from build123d import *

# Parameters (mm, degrees)
SKETCH_1_W          = 720
SKETCH_1_H          = 110
SKETCH_1_R          = 5
EXTRUDE_1_DEPTH     = 2
SKETCH_2_W          = 720
SKETCH_2_H          = 3
EXTRUDE_2_DEPTH     = 20
SKETCH_3_R          = 2.5
CUT_EXTRUDE_3_DEPTH = 114


with BuildPart() as part:
    # 草图1 → 凸台-拉伸1 (new body)
    with BuildSketch(Plane.XY):
        with Locations((266.780748393, 19.519407272)):
            Rectangle(SKETCH_1_W, SKETCH_1_H)
        with Locations((0, -5.480592728)):
            Circle(SKETCH_1_R, mode=Mode.SUBTRACT)
        with Locations((179.094970205, -5.480592728)):
            Circle(SKETCH_1_R, mode=Mode.SUBTRACT)
        with Locations((354.466526581, -5.480592728)):
            Circle(SKETCH_1_R, mode=Mode.SUBTRACT)
        with Locations((529.466526581, -5.480592728)):
            Circle(SKETCH_1_R, mode=Mode.SUBTRACT)
    extrude(amount=EXTRUDE_1_DEPTH)

    # 草图2 → 凸台-拉伸2 (add)
    with BuildSketch(Plane.XY.offset(2)):
        with Locations((266.780748393, 73.019407272)):
            Rectangle(SKETCH_2_W, SKETCH_2_H)
        with Locations((266.780748393, -33.980592728)):
            Rectangle(SKETCH_2_W, SKETCH_2_H)
    extrude(amount=EXTRUDE_2_DEPTH)

    # 草图3 → 切除-拉伸3 (cut)
    with BuildSketch(Plane(origin=(0, 74.519407272, 0), x_dir=(1, 0, 0), z_dir=(0, 1, 0))):
        with Locations(Location((456.780748393, -12, 0), (0, 0, 270))):
            Circle(SKETCH_3_R)
        with Locations(Location((616.780748393, -12, 0), (0, 0, 270))):
            Circle(SKETCH_3_R)
        with Locations(Location((436.780748393, -12, 0), (0, 0, 270))):
            Circle(SKETCH_3_R)
        with Locations(Location((276.780748393, -12, 0), (0, 0, 270))):
            Circle(SKETCH_3_R)
        with Locations(Location((256.780748393, -12, 0), (0, 0, 270))):
            Circle(SKETCH_3_R)
        with Locations(Location((96.780748393, -12, 0), (0, 0, 270))):
            Circle(SKETCH_3_R)
        with Locations(Location((76.780748393, -12, 0), (0, 0, 270))):
            Circle(SKETCH_3_R)
        with Locations(Location((-83.219251607, -12, 0), (0, 0, 270))):
            Circle(SKETCH_3_R)
    extrude(amount=-CUT_EXTRUDE_3_DEPTH, mode=Mode.SUBTRACT)


solid = part.part
Here's how the part is built. I have some questions about the finished solid (model axes, mm). A direction names the side the tool comes from. Give positions to 0.01 mm unless a question says otherwise; leave off trailing zeros. Loops run counter-clockwise (first coordinate to the right, second up) from the corner with the lowest first, then second, coordinate; pieces in that order, holes last. Notation, with made-up numbers: (65.25, 3.5) -> (76.25, 3.5) arc R31 cw to (76.25, 40.5) -> close; hole circle Ø4 at (42.5, 89.5). An arc over 180 degrees is marked (long way). One line per item, written item: value.
Q1. I'm going to push flat-ended pins straight in: pin 1 Ø1.5 at (x, y) = (346, 37.5) entering from -Z; pin 2 Ø3 at (x, z) = (456.78, 12) entering from -Y; pin 3 Ø1.5 at (x, y) = (550, -0.5) entering from +Z. Where does each tip first touch, or does it pass through?
Answers follow:
pin 1: z = 0
pin 2: through
pin 3: z = 2
Q2. If I drill on line 1 along Y through (x, z) = (393.5, 10); line 2 along Z through (x, y) = (-16, -15.5), over which ranges is the centre line in solid material (lowest first)?
Answers follow:
line 1: -35.48 to -32.48, 71.52 to 74.52
line 2: 0 to 2
Q3. Suppose I cut it at B-B on y = 60.5. Please give me the cut outline in (x, z).
Answers follow:
outline: (-93.22, 0) -> (626.78, 0) -> (626.78, 2) -> (-93.22, 2) -> close
Q4. On a 3-axis mill with a long thin cutter (end or side, diameter ignored), from which of +Z, -Z, +X, -X, +Y, -Y can I reach the whole of each face in a straight line? I mean faces 1 (the face through (262, -35.481, 11)), 2 (the face through (262, -32.481, 12)). Say none if no direction works.
Answers follow:
face 1: +Z, -Z, +X, -X, -Y
face 2: +Z, +X, -X
Q5. Suppose I cut it at A-A on x = 470.5. Please give me the cut outline in (y, z), then the cut area to 3 significant figures.
Answers follow:
outline: (-35.48, 0) -> (74.52, 0) -> (74.52, 22) -> (71.52, 22) -> (71.52, 2) -> (-32.48, 2) -> (-32.48, 22) -> (-35.48, 22) -> close
area: 340 mm^2
